Can you work these out from the model? Positions are in its coordinate system, mm. Coordinates: 2 decimals unless noted, no trailing zeros. Loops run counter-clockwise (first coordinate to the right, second up) from the corner with the lowest first, then second, coordinate; pieces in that order, holes last.
```python
from build123d import *

# Parameters (mm, degrees)
SKETCH_1_R      = 1.6
EXTRUDE_1_DEPTH = 3
FILLET_1_R      = 10


with BuildPart() as part:
    # 草图1 → 凸台-拉伸1 (new body)
    with BuildSketch(Plane.XY):
        Polygon((33.75, 17.5), (48.75, 17.5), (48.75, -17.5), (33.75, -17.5), (-33.75, -17.5), (-33.75, 17.5), align=None)
        with Locations((-26.25, 10)):
            Circle(SKETCH_1_R, mode=Mode.SUBTRACT)
        with Locations((-26.25, -10)):
            Circle(SKETCH_1_R, mode=Mode.SUBTRACT)
        with Locations((26.25, -10)):
            Circle(SKETCH_1_R, mode=Mode.SUBTRACT)
        with Locations((26.25, 10)):
            Circle(SKETCH_1_R, mode=Mode.SUBTRACT)
    extrude(amount=EXTRUDE_1_DEPTH)

    # 圆角1
    fillet_1_edges = [part.edges().sort_by_distance(p)[0] for p in [
        (48.75, 17.5, 1.5),
        (48.75, -17.5, 1.5),
        (-33.75, -17.5, 1.5),
        (-33.75, 17.5, 1.5),
    ]]
    fillet(fillet_1_edges, radius=FILLET_1_R)


solid = part.part
```
(1) I want a section at B-B on z = 1.9. Write out the boundary of the cut face in (x, y), then the cut area to 3 significant figures.
Check values:
outline: (-33.75, -7.5) arc R10 ccw to (-23.75, -17.5) - (38.75, -17.5) arc R10 ccw to (48.75, -7.5) - (48.75, 7.5) arc R10 ccw to (38.75, 17.5) - (-23.75, 17.5) arc R10 ccw to (-33.75, 7.5) - close; hole circle Ø3.2 at (-26.25, -10); hole circle Ø3.2 at (-26.25, 10); hole circle Ø3.2 at (26.25, -10); hole circle Ø3.2 at (26.25, 10)
area: 2,770 mm2
(2) If I drill on probe 1 along Y at (x, z) = (26.25, 0.9); probe 2 along Y at (x, z) = (-26.25, 1.05); probe 3 along X at (y, z) = (-10.5, 0.6), over which ranges is the centre line in solid material (lowest first)?
Check values:
probe 1: y = -17.5 to -11.6, -8.4 to 8.4, 11.6 to 17.5
probe 2: y = -17.18 to -11.6, -8.4 to 8.4, 11.6 to 17.18
probe 3: x = -33.29 to -27.77, -24.73 to 24.73, 27.77 to 48.29
(3) I want a section at C-C on y = 10. Write out the boundary of the cut face in (x, z).
Check values:
outline: (-33.43, 0) - (-27.85, 0) - (-27.85, 3) - (-33.43, 3) - close; (-24.65, 0) - (24.65, 0) - (24.65, 3) - (-24.65, 3) - close; (27.85, 0) - (48.43, 0) - (48.43, 3) - (27.85, 3) - close
(4) I want a section at A-A on x = 26.25. Write out the boundary of the cut face in (y, z), then the cut area to 3 significant figures.
Check values:
outline: (-17.5, 0) - (-11.6, 0) - (-11.6, 3) - (-17.5, 3) - close; (-8.4, 0) - (8.4, 0) - (8.4, 3) - (-8.4, 3) - close; (11.6, 0) - (17.5, 0) - (17.5, 3) - (11.6, 3) - close
area: 85.8 mm2
(5) I want a section at D-D on x = 41.5. Write out the boundary of the cut face in (y, z), then the cut area to 3 significant figures.
Check values:
outline: (-17.11, 0) - (17.11, 0) - (17.11, 3) - (-17.11, 3) - close
area: 103 mm2
(6) I'm going to push flat-ended pins straight in: pin 1 (4 mm diameter, centred on x = 26.25, y = 10, fed in from +Z); pin 2 (1.9 mm diameter, centred on x = -26.25, y = -10, fed in from +Z); pin 3 (1 mm diameter, centred on y = -9, z = 0.5, fed in from +X). Where does each tip first touch, or does it pass through?
Check values:
pin 1: stops at z = 3
pin 2: passes through
pin 3: stops at x = 48.7
(7) If we mould it in two halves opening along Y, with no side actions, what happens to faces 1 (the flat face through (7, -17.5, 1)), 2 (the cylindrical face through (-30.74, 14.65, 1.52)), 3 (the flat face through (-33.75, 0, 1)), 4 (the cylindrical face through (-26.6, -11.56, 1.48))? For each: released by +Y, released by -Y, zero draft, split by the parting line, or undercut.
Check values:
face 1: released by -Y
face 2: released by +Y
face 3: zero draft
face 4: undercut
